Source: CAD feature listing. Evaluate the final solid. Frame: model axes, mm. A direction names the side the tool comes from. Give positions to 0.01 mm unless a question says otherwise; leave off trailing zeros. Order: outer loops, then holes, each group sorted by start corner. A loop starts at its lowest first (then second) coordinate and runs counter-clockwise, first axis right, second up. Notation, with made-up numbers: M 56,55.25 L 68,55.25 A16 ccw 68,59.25 Z; hole C 32.25,19 d7. An arc over 180 degrees is marked long. Return JSON: item names as keys, results as strings.
from build123d import *

# Parameters (mm, degrees)
F0_R     = 88.9
F1_DEPTH = 152.4
F4_DEPTH = 152.401
F5_DEPTH = 152.401


with BuildPart() as f1:
    # F0 (on Front) → F1 (new body)
    with BuildSketch(Plane.XZ):
        Circle(F0_R)
    extrude(amount=-F1_DEPTH)

    # F3 (on face) → F4 (cut, through all)
    with BuildSketch(Plane.XZ):
        with BuildLine():
            ThreePointArc((6.345302, 82.305769), (0, 76.2), (-6.345302, 82.305769))
            ThreePointArc((-6.345302, 82.305769), (-58.371665, 58.371665), (-82.305769, 6.345302))
            ThreePointArc((-82.305769, 6.345302), (-77.974338, 4.402933), (-76.2, 0))
            ThreePointArc((-76.2, 0), (-77.974338, -4.402933), (-82.305769, -6.345302))
            ThreePointArc((-82.305769, -6.345302), (-58.371665, -58.371665), (-6.345302, -82.305769))
            ThreePointArc((-6.345302, -82.305769), (0, -76.2), (6.345302, -82.305769))
            ThreePointArc((6.345302, -82.305769), (58.371665, -58.371665), (82.305769, -6.345302))
            ThreePointArc((82.305769, -6.345302), (76.2, 0), (82.305769, 6.345302))
            ThreePointArc((82.305769, 6.345302), (58.371665, 58.371665), (6.345302, 82.305769))
        make_face()
    extrude(amount=-F4_DEPTH, mode=Mode.SUBTRACT)

    # F2 (on face) → F5 (cut, through all)
    with BuildSketch(Plane.XZ):
        with BuildLine():
            ThreePointArc((-2.7936, 82.502717), (-1.958868, 80.557697), (0, 79.756))
            ThreePointArc((0, 79.756), (1.958868, 80.557697), (2.7936, 82.502717))
            ThreePointArc((2.7936, 82.502717), (2.7939, 82.526358), (2.794, 82.55))
            ThreePointArc((2.794, 82.55), (-0.023642, 85.3439), (-2.7936, 82.502717))
        make_face()
        with BuildLine():
            ThreePointArc((-82.502717, 2.7936), (-85.344, 0), (-82.502717, -2.7936))
            ThreePointArc((-82.502717, -2.7936), (-80.557697, -1.958868), (-79.756, 0))
            ThreePointArc((-79.756, 0), (-80.557697, 1.958868), (-82.502717, 2.7936))
        make_face()
        with BuildLine():
            ThreePointArc((79.756, 0), (80.557697, -1.958868), (82.502717, -2.7936))
            ThreePointArc((82.502717, -2.7936), (84.508868, -1.992303), (85.344, 0))
            ThreePointArc((85.344, 0), (84.508868, 1.992303), (82.502717, 2.7936))
            ThreePointArc((82.502717, 2.7936), (80.557697, 1.958868), (79.756, 0))
        make_face()
        with BuildLine():
            ThreePointArc((2.794, -82.55), (2.7939, -82.526358), (2.7936, -82.502717))
            ThreePointArc((2.7936, -82.502717), (1.958868, -80.557697), (0, -79.756))
            ThreePointArc((0, -79.756), (-1.958868, -80.557697), (-2.7936, -82.502717))
            ThreePointArc((-2.7936, -82.502717), (-0.023642, -85.3439), (2.794, -82.55))
        make_face()
    extrude(amount=-F5_DEPTH, mode=Mode.SUBTRACT)


solid = f1.part
1. Draft query along X for faces 3 (the face through (57.79, 75.13, -58.95)), 4 (the face through (84.795, 75.133, 26.703)), 5 (the face through (0, 0, -79)). Return one class per face: pulls with the +X half, pulls with the -X half, needs draft (parallel to the pull), parting line crosses it, or undercut.
Evaluation:
{"face 3": "undercut", "face 4": "parting line crosses it", "face 5": "needs draft"}
2. Set-up query: faces 1 (the face through (58.95, 75.13, 57.79)), 2 (the face through (0, 152.4, -79)). Return all of +Z, -Z, +X, -X, +Y, -Y with unobstructed straight access to the full face (end or side cutting, diameter ignored); none if empty.
Evaluation:
{"face 1": "+Y, -Y", "face 2": "+Z, -Z, +X, -X, +Y"}
3. Ray query, probe 1 along X at (y, z) = (59, -64); probe 2 along Z at (x, y) = (-72.5, 95.5); probe 3 along Z at (x, y) = (-55.5, 112.5). Return the intervals inside material, ascending.
Evaluation:
{"probe 1": "x = -61.7 to -52.14, 52.14 to 61.7", "probe 2": "z = -51.45 to -39.47, 39.47 to 51.45", "probe 3": "z = -69.45 to -61.11, 61.11 to 69.45"}
4. Section query A-A (y = 98). Return loops of the section in (x, z), then the cut area to 3 significant figures.
Evaluation:
{"outline": "C 0,0 d177.8; hole C -82.55,0 d5.59; hole M -82.31,-6.35 A82.55 ccw -6.35,-82.31 A6.35 cw 6.35,-82.31 A82.55 ccw 82.31,-6.35 A6.35 cw 82.31,6.35 A82.55 ccw 6.35,82.31 A6.35 cw -6.35,82.31 A82.55 ccw -82.31,6.35 A6.35 cw Z; hole M 2.79,-82.55 A2.79 ccw 2.79,-82.5 A2.79 ccw long Z; hole M 2.79,82.5 A2.79 ccw 2.79,82.55 A2.79 ccw long Z; hole M 82.5,-2.79 A2.79 ccw long 82.5,2.79 A2.79 ccw Z", "area": "3,570 mm^2"}
5. First-contact query: pin 1 (4 mm diameter, centred on x = -21, y = 56.5, fed in from +Z); pin 2 (4 mm diameter, centred on y = 26.5, z = 48.5, fed in from +X); pin 3 (1 mm diameter, centred on x = 9.5, y = 98, fed in from -Z). Flat tips, straight axial feed; report the tip coordinate or a pass-through.
Evaluation:
{"pin 1": "stops at z = 86.85", "pin 2": "stops at x = 75.77", "pin 3": "stops at z = -88.44"}
6. Section query B-B (x = 64). Return loops of the section in (y, z).
Evaluation:
{"outline": "M 0,-61.7 L 152.4,-61.7 L 152.4,-52.14 L 0,-52.14 Z; M 0,52.14 L 152.4,52.14 L 152.4,61.7 L 0,61.7 Z"}
7. Section query C-C (z = 10.5). Return loops of the section in (x, y), then the cut area to 3 significant figures.
Evaluation:
{"outline": "M -88.28,0 L -81.88,0 L -81.88,152.4 L -88.28,152.4 Z; M 81.88,0 L 88.28,0 L 88.28,152.4 L 81.88,152.4 Z", "area": "1,950 mm^2"}
